The model under review builds one solid part; all positions refer to its coordinate system, in mm. A direction names the side the tool comes from. Round coordinates to 2 decimals unless told otherwise and drop trailing zeros. Loops run counter-clockwise (first coordinate to the right, second up) from the corner with the lowest first, then second, coordinate; pieces in that order, holes last. Notation, with made-up numbers: M -32.75,7 L -2.75,7 A28 cw -2.75,45 Z; hole C -19.5,32 d1. An arc over 180 degrees is marked long. Answer in a Markdown table with one row per item. Add a question column.
Autodesk Inventor part; units mm, degrees
ref_plane "YZ Plane" through (0, 0, 0) normal (1, 0, 0) x (0, 1, 0)
ref_plane "XZ Plane" through (0, 0, 0) normal (0, 1, 0) x (-1, 0, 0)
ref_plane "XY Plane" through (0, 0, 0) normal (0, 0, 1) x (1, 0, 0)
sketch "Sketch1" plane through (0, 0, 0) normal (0, 0, 1) x (1, 0, 0)
  circle A0 centre (0, 0) radius 2.0828
  dimension "d0" = 4.1656
extrude "Extrusion1" add sketch "Sketch1" along normal blind 12.7
sketch "Sketch2" plane through (0, 0, 0) normal (0, 1, 0) x (-1, 0, 0)
  line L0 (0, 0) -> (0, -2.2098)
  line L1 (0, 0) -> (3.9624, 0)
  line L2 (0, -2.2098) -> (2.032, -2.2098)
  line L3 (3.9624, 0) -> (3.9624, 3.6562) construction
  arc A0 (2.032, -2.2098) -> (3.9624, -0.4599) centre (0.1837, 1.7689) ccw
  line L4 (4.5847, 0.6553) -> (4.5847, -0.2608) construction
  line L5 (3.9624, -0.4599) -> (3.9624, 0)
  dimension "d3" = 2.2098
  dimension "d6" = 2.032
  dimension "d19" = 3.9624
revolve "Revolution1" add sketch "Sketch2" angle 360 about axis through (0, 0, 0) along (0, 0, -1)
sketch "Sketch3" plane through (0, 0, -2.2098) normal (0, 0, -1) x (-1, 0, 0)
  circle A0 centre (0, 0) radius 2.032
  line L0 (-0.6874, 1.1906) -> (0.6874, 1.1906)
  line L1 (0.6874, 1.1906) -> (1.3748, 0)
  line L2 (1.3748, 0) -> (0.6874, -1.1906)
  line L3 (0.6874, -1.1906) -> (-0.6874, -1.1906)
  line L4 (-0.6874, -1.1906) -> (-1.3748, 0)
  line L5 (-1.3748, 0) -> (-0.6874, 1.1906)
  dimension "d8" = 2.3813
extrude "Extrusion2" cut sketch "Sketch3" against normal blind 1.5875 contours L0 L1 L2 L3 L4 L5
chamfer "Chamfer1" distance 0.508 angle 45 1 edges at (-2.0828, 0, 12.7)
thread "Thread1"
properties part number "10-32 x500 button head" material "Steel"
1. To check wall thickness, follow probe 1 along Y at (x, z) = (0, 11); probe 2 along Z at (x, y) = (0.5, 0.25); probe 3 along X at (y, z) = (0.75, 10.75). State the ranges of each line that lie inside material, in increasing order.
2. For pin 1 Ø3 at (y, z) = (1.5, 3.5) entering from -X; pin 2 Ø1.5 at (x, z) = (2.5, 11) entering from -Y; pin 3 Ø1 at (x, y) = (-2.5, -1.5) entering from +Z, all flat-tipped, find the tip position at first contact; note any pin that passes through.
3. Take a section at A-A, the plane z = 6.5. State the section outline as (x, y) points.
4. Machinability: for faces 1 (the flat face through (-1, -1, -2.21)), 2 (the flat face through (-1.036, -0.587, -1.427)), 3 (the flat face through (-2, -2, 0)), which of the approach directions +Z, -Z, +X, -X, +Y, -Y give a long, thin tool a straight path to every point of the face, cutting with its end or side? Answer none if there is none.
Check sheet entries:
| question | item | result |
|---|---|---|
| 1 | probe 1 | y = -2.08 to 2.08 |
| 1 | probe 2 | z = -0.62 to 12.7 |
| 1 | probe 3 | x = -1.94 to 1.94 |
| 2 | pin 1 | stops at x = -2.08 |
| 2 | pin 2 | stops at y = -1.13 |
| 2 | pin 3 | stops at z = 0 |
| 3 | outline | C 0,0 d4.17 |
| 4 | face 1 | -Z, +X, -X, +Y, -Y |
| 4 | face 2 | -Z |
| 4 | face 3 | +Z |
